Here's how the part is built. I have some questions about the finished solid (model axes, mm). Round coordinates to 2 decimals unless told otherwise and drop trailing zeros. Write each loop counter-clockwise with the first axis right and the second up, starting at its lowest first coordinate (ties: lowest second). Pieces come first, ordered by that corner, then holes. Notation, with made-up numbers: (-7.75, -9.75) - (38.25, -9.75) arc R13 cw to (38.25, -2.75) - close; hole circle Ø7 at (-3, 61.25). An arc over 180 degrees is marked (long way). Return JSON: item names as keys, results as strings. Group by question number.
Autodesk Inventor part; units mm, degrees
ref_plane "YZ Plane" through (0, 0, 0) normal (1, 0, 0) x (0, 1, 0)
ref_plane "XZ Plane" through (0, 0, 0) normal (0, 1, 0) x (-1, 0, 0)
ref_plane "XY Plane" through (0, 0, 0) normal (0, 0, 1) x (1, 0, 0)
sketch "Эскиз1" plane through (0, 0, 0) normal (0, 1, 0) x (-1, 0, 0)
  circle A0 centre (0, 0) radius 58.5
  line L0 (40, -37.5) -> (-40, -37.5) construction
  line L1 (-40, -37.5) -> (-40, 37.5) construction
  line L2 (-40, 37.5) -> (40, 37.5) construction
  line L3 (40, 37.5) -> (40, -37.5) construction
  line L4 (40, -37.5) -> (-40, 37.5) construction
  line L5 (-40, -37.5) -> (40, 37.5) construction
  line L6 (-42.6779, -40.0106) -> (42.6779, -40.0106)
  line L7 (42.6779, -40.0106) -> (42.6779, 40.0106)
  line L8 (42.6779, 40.0106) -> (-42.6779, 40.0106)
  line L9 (-42.6779, 40.0106) -> (-42.6779, -40.0106)
  line L10 (-42.6779, -40.0106) -> (42.6779, 40.0106) construction
  line L11 (42.6779, -40.0106) -> (-42.6779, 40.0106) construction
  arc A1 (25.026, 40.0106) -> (27.4557, 49.3805) centre (25.026, 45.0106) ccw
  circle A2 centre (0, 0) radius 56.5
  arc A3 (-27.4557, 49.3805) -> (-25.026, 40.0106) centre (-25.026, 45.0106) ccw
  arc A4 (52.3069, 21.3599) -> (42.6779, 19.4696) centre (47.6779, 19.4696) ccw
  arc A5 (42.6779, -19.4696) -> (52.3069, -21.3599) centre (47.6779, -19.4696) ccw
  arc A6 (27.4557, -49.3805) -> (25.026, -40.0106) centre (25.026, -45.0106) ccw
  arc A7 (-25.026, -40.0106) -> (-27.4557, -49.3805) centre (-25.026, -45.0106) ccw
  arc A8 (-52.3069, -21.3599) -> (-42.6779, -19.4696) centre (-47.6779, -19.4696) ccw
  arc A9 (-42.6779, 19.4696) -> (-52.3069, 21.3599) centre (-47.6779, 19.4696) ccw
  dimension "d0" = 117
  dimension "d3" = 113
  dimension "d1" = 80
  dimension "d2" = 75
  dimension "d4" = 10
  dimension "d5" = 10
  dimension "d6" = 10
  dimension "d7" = 10
  dimension "d8" = 10
  dimension "d9" = 10
  dimension "d10" = 10
  dimension "d11" = 10
extrude "Выдавливание1" add sketch "Эскиз1" along normal blind 2 contours A0 L7 A2 | L8 A2 A0 | L7 A2 L8 | A0 L6 A2 | L6 A2 L7 | L9 A2 A0 | L8 A2 L9 | A2 A4 L7 | L7 A2 L6 L9 L8 | L8 A1 A2 | L9 A2 L6 | A2 A6 L6 | L7 A5 A2 | A2 A3 L8 | L9 A9 A2 | L6 A7 A2 | A2 A8 L9
properties part number "InnerCap"
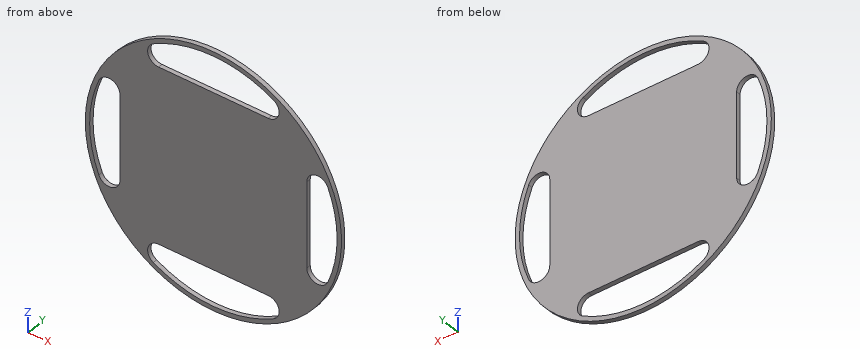
1) Will these pins go through, and if not, where does the flat tip stop? pin 1 Ø0.6 at (y, z) = (1, -6) entering from -X; pin 2 Ø0.6 at (x, y) = (-8, 1) entering from +Z.
2) I need wall thicknesses on line 1 along X through (y, z) = (0.7, -19); line 2 along Z through (x, y) = (3, 1.2); line 3 along Z through (x, y) = (-11, 0.5). Which ranges of each line are inside material? Lowest first, please.
3) Imagine slicing it at B-B (x = 14). Please give me the cut outline in (y, z), plus the area to 3 significant figures.
4) Imagine slicing it at A-A (z = 0). Please give me the cut outline in (x, y), plus the area to 3 significant figures.
5) Imagine slicing it at C-C (x = -50.5). Please give me the cut outline in (y, z).
6) Imagine slicing it at D-D (y = 0.95). Please give me the cut outline in (x, z), plus the area to 3 significant figures.
Results found:
{
 "1": {"pin 1": "stops at x = -58.22", "pin 2": "stops at z = 57.99"},
 "2": {"line 1": "x = -55.33 to -53.21, -42.68 to 42.68, 53.21 to 55.33", "line 2": "z = -58.42 to -56.42, -40.01 to 40.01, 56.42 to 58.42", "line 3": "z = -57.46 to -55.42, -40.01 to 40.01, 55.42 to 57.46"},
 "3": {"outline": "(0, -56.8) - (2, -56.8) - (2, -54.74) - (0, -54.74) - close; (0, -40.01) - (2, -40.01) - (2, 40.01) - (0, 40.01) - close; (0, 54.74) - (2, 54.74) - (2, 56.8) - (0, 56.8) - close", "area": "168 mm²"},
 "4": {"outline": "(-58.5, 0) - (-56.5, 0) - (-56.5, 2) - (-58.5, 2) - close; (-42.68, 0) - (42.68, 0) - (42.68, 2) - (-42.68, 2) - close; (56.5, 0) - (58.5, 0) - (58.5, 2) - (56.5, 2) - close", "area": "179 mm²"},
 "5": {"outline": "(0, -29.53) - (2, -29.53) - (2, -23.6) - (0, -23.6) - close; (0, 23.6) - (2, 23.6) - (2, 29.53) - (0, 29.53) - close"},
 "6": {"outline": "circle Ø117 at (0, 0); hole (-52.31, -21.36) arc R5 ccw to (-42.68, -19.47) - (-42.68, 19.47) arc R5 ccw to (-52.31, 21.36) arc R56.5 ccw to start; hole (-27.46, -49.38) arc R56.5 ccw to (27.46, -49.38) arc R5 ccw to (25.03, -40.01) - (-25.03, -40.01) arc R5 ccw to start; hole (-27.46, 49.38) arc R5 ccw to (-25.03, 40.01) - (25.03, 40.01) arc R5 ccw to (27.46, 49.38) arc R56.5 ccw to start; hole (42.68, -19.47) arc R5 ccw to (52.31, -21.36) arc R56.5 ccw to (52.31, 21.36) arc R5 ccw to (42.68, 19.47) - close", "area": "7,990 mm²"}
}
